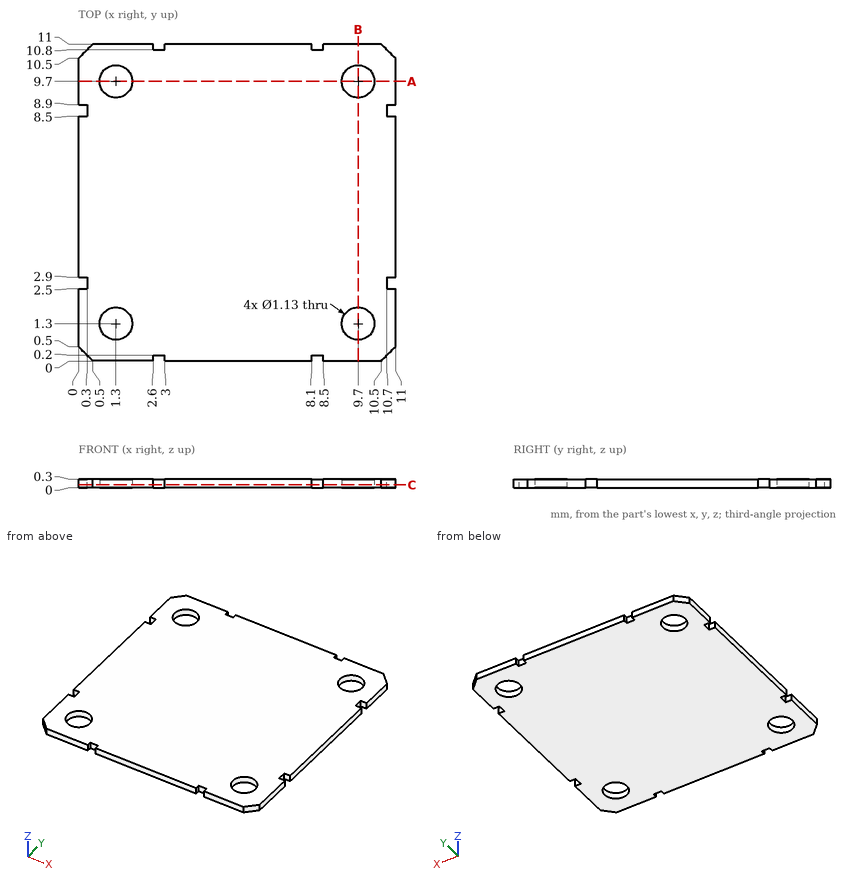
Design review of the part shown in the three views and the two pictorial views. Dimensions are in mm from the part's minimum x, y and z. Round coordinates to 2 decimals unless told otherwise and drop trailing zeros. Loops run counter-clockwise (first coordinate to the right, second up) from the corner with the lowest first, then second, coordinate; pieces in that order, holes last. Notation, with made-up numbers: (-11, -13) - (16, -13) arc R24 cw to (16, 2) - close; hole circle Ø5 at (-20.5, -16.75). An arc over 180 degrees is marked (long way). Use CSV: the item, a comma, the result in double quotes.
(1) For line 1 (X direction, y = 1.3, z = 0.1) (3 decimals); line 2 (X direction, y = 9.5, z = 0.05); line 3 (X direction, y = 8.75, z = 0.2), list the stretches that pass through material, from the lowest coordinate up.
Working result:
line 1,"x = 0 to 0.735, 1.865 to 9.135, 10.265 to 11"
line 2,"x = 0 to 0.77, 1.83 to 9.17, 10.23 to 11"
line 3,"x = 0.3 to 10.7"
(2) Take a section at A-A, the plane y = 9.7. Give the boundary of the cut face in (x, z) (3 decimals).
Working result:
outline,"(0, 0) - (0.735, 0) - (0.735, 0.3) - (0, 0.3) - close; (1.865, 0) - (9.135, 0) - (9.135, 0.3) - (1.865, 0.3) - close; (10.265, 0) - (11, 0) - (11, 0.3) - (10.265, 0.3) - close"
(3) Take a section at C-C, the plane z = 0.1. State how many separate pieces and enclosed holes the cut face has, plus the area to 3 significant figures.
Working result:
separate pieces,"1"
enclosed holes,"4"
area,"116 mm^2"
